Build history of the part. All positions in model axes, mm. A direction names the side the tool comes from. Round coordinates to 2 decimals unless told otherwise and drop trailing zeros. Loops run counter-clockwise (first coordinate to the right, second up) from the corner with the lowest first, then second, coordinate; pieces in that order, holes last. Notation, with made-up numbers: (45, 38.25) - (81, 38.25) arc R7 ccw to (81, 51.25) - close; hole circle Ø4 at (-12.75, -7.5). An arc over 180 degrees is marked (long way). Use one line per item in the form item = value. Start each with the question number.
Q1. Saw through at A-A (z = 7.25). Give the cut face in (x, y), then the cut area to 3 significant figures.
Q2. Pin check, flat tip, straight feed: pin 1 (10.5 mm diameter, centred on x = 180.95, y = -125, fed in from -Z). Stop position of the tip, or through.
Q3. Drill centre lines: line 1 (Y direction, x = 180.95, z = 5.25); line 2 (X direction, y = -74.5, z = 9.5); line 3 (X direction, y = -122.5, z = 9.5). Where is each one in solid material? Low to high.
Q4. 3-axis set-ups, long thin cutter, end or side, ignore diameter. For faces 4 (the face through (-206.35, 2, 6)), 5 (the face through (14.855, -95.169, 6.261)): which of +Z, -Z, +X, -X, +Y, -Y reach the whole face in a straight line?
Q5. Mould opens along X. For faces 1 (the face through (206.35, -2, 6)), 2 (the face through (3, 150, 6)), 3 (the face through (-14.86, -125.56, 6.26)) say: released by +X, released by -X, zero draft, split by the parting line, or undercut.
```python
from build123d import *

# Parameters (mm, degrees)
SKETCH1_R           = 4
BOSS_EXTRUDE2_DEPTH = 12.7
CUT_EXTRUDE1_REACH  = 257.424
SKETCH2_R           = 4
FILLET1_R           = 4


with BuildPart() as part:
    # Sketch1 → Boss-Extrude2 (new body)
    with BuildSketch(Plane.XY):
        Polygon((-187.3, -150), (187.3, -150), (206.35, -150), (206.35, 150), (187.3, 150), (-187.3, 150), (-206.35, 150), (-206.35, -150), align=None)
        Polygon((14.318912319, -137.41311332), (8.66205807, -131.75625907), (0, -140.41831714), (-30.0520382, -110.366278939), (0, -80.314240739), (30.0520382, -110.366278939), (21.389980131, -119.028337009), (27.04683438, -124.685191258), align=None, mode=Mode.SUBTRACT)
        with Locations((-20.590065585, -87.466385575)):
            Circle(SKETCH1_R, mode=Mode.SUBTRACT)
        with Locations((20.590065585, -87.466385575)):
            Circle(SKETCH1_R, mode=Mode.SUBTRACT)
    extrude(amount=BOSS_EXTRUDE2_DEPTH)

    # Sketch2 → Cut-Extrude1 (cut, up to next)
    with BuildSketch(Plane.XY.offset(12.7), mode=Mode.PRIVATE) as cut_extrude1_sk1:
        with Locations((-180.95, -75)):
            Circle(SKETCH2_R)
    cut_extrude1_tool1 = extrude(cut_extrude1_sk1.sketch, amount=-CUT_EXTRUDE1_REACH, mode=Mode.PRIVATE) & part.part
    # Sketch2 → Cut-Extrude1 (cut, up to next)
    with BuildSketch(Plane.XY.offset(12.7), mode=Mode.PRIVATE) as cut_extrude1_sk2:
        with Locations((-180.95, -125)):
            Circle(SKETCH2_R)
    cut_extrude1_tool2 = extrude(cut_extrude1_sk2.sketch, amount=-CUT_EXTRUDE1_REACH, mode=Mode.PRIVATE) & part.part
    # Sketch2 → Cut-Extrude1 (cut, up to next)
    with BuildSketch(Plane.XY.offset(12.7), mode=Mode.PRIVATE) as cut_extrude1_sk3:
        with Locations((180.95, -125)):
            Circle(SKETCH2_R)
    cut_extrude1_tool3 = extrude(cut_extrude1_sk3.sketch, amount=-CUT_EXTRUDE1_REACH, mode=Mode.PRIVATE) & part.part
    # Sketch2 → Cut-Extrude1 (cut, up to next)
    with BuildSketch(Plane.XY.offset(12.7), mode=Mode.PRIVATE) as cut_extrude1_sk4:
        with Locations((180.95, -75)):
            Circle(SKETCH2_R)
    cut_extrude1_tool4 = extrude(cut_extrude1_sk4.sketch, amount=-CUT_EXTRUDE1_REACH, mode=Mode.PRIVATE) & part.part
    add(cut_extrude1_tool1.solids().sort_by_distance((-180.95, -75, 12.7))[0], mode=Mode.SUBTRACT)
    add(cut_extrude1_tool2.solids().sort_by_distance((-180.95, -125, 12.7))[0], mode=Mode.SUBTRACT)
    add(cut_extrude1_tool3.solids().sort_by_distance((180.95, -125, 12.7))[0], mode=Mode.SUBTRACT)
    add(cut_extrude1_tool4.solids().sort_by_distance((180.95, -75, 12.7))[0], mode=Mode.SUBTRACT)

    # Fillet1
    fillet1_edges = [part.edges().sort_by_distance(p)[0] for p in [
        (0, -80.314240739, 6.35),
        (-30.0520382, -110.366278939, 6.35),
        (0, -140.41831714, 6.35),
        (14.318912319, -137.41311332, 6.35),
        (27.04683438, -124.685191258, 6.35),
        (30.0520382, -110.366278939, 6.35),
    ]]
    fillet(fillet1_edges, radius=FILLET1_R)


solid = part.part
```
Report:
q1.outline = (-206.35, -150) - (206.35, -150) - (206.35, 150) - (-206.35, 150) - close; hole circle Ø8 at (-180.95, -125); hole circle Ø8 at (-180.95, -75); hole (-27.22, -113.19) - (-2.83, -137.59) arc R4 ccw to (2.83, -137.59) - (8.66, -131.76) - (11.49, -134.58) arc R4 ccw to (17.15, -134.58) - (24.22, -127.51) arc R4 ccw to (24.22, -121.86) - (21.39, -119.03) - (27.22, -113.19) arc R4 ccw to (27.22, -107.54) - (2.83, -83.14) arc R4 ccw to (-2.83, -83.14) - (-27.22, -107.54) arc R4 ccw to start; hole circle Ø8 at (-20.59, -87.47); hole circle Ø8 at (20.59, -87.47); hole circle Ø8 at (180.95, -125); hole circle Ø8 at (180.95, -75)
q1.area = 122,000 mm²
q2.pin_1 = 0
q3.line_1 = -150 to -129, -121 to -79, -71 to 150
q3.line_2 = -206.35 to -184.92, -176.98 to 176.98, 184.92 to 206.35
q3.line_3 = -206.35 to -184.07, -177.83 to -17.92, 24.74 to 177.83, 184.07 to 206.35
q4.face_4 = +Z, -Z, -X, +Y, -Y
q4.face_5 = +Z, -Z
q5.face_1 = released by +X
q5.face_2 = zero draft
q5.face_3 = undercut
